Model file for the job. Use its own axes, mm. A direction names the side the tool comes from. Coordinates: 2 decimals unless noted, no trailing zeros. Put each result on its own line as item: value. Start each with the question number.
Q1. Drill centre lines: line 1 along Y through (x, z) = (12, 0.2); line 2 along Y through (x, z) = (-16, 1.3); line 3 along Z through (x, y) = (3, 4) (3 decimals). Where is each one in solid material? Low to high.
Q2. Cut at A-A (x = 0). Give the number of separate pieces and of enclosed holes in the cut face, then the cut area to 3 significant figures.
Q3. Drop flat-ended pins along their axis: pin 1 (0.9 mm diameter, centred on x = 0, y = 14.605, fed in from -Z); pin 2 (1.5 mm diameter, centred on y = -9, z = 0.5, fed in from +X); pin 3 (2 mm diameter, centred on x = 0, y = 6.985, fed in from -Z); pin 4 (5 mm diameter, centred on x = 6, y = 6.5, fed in from +Z) (3 decimals). Give the stop position or say it passes through.
Q4. Pull direction Y, two halves, no side cores. Call faces 6 (the cylindrical face through (-6.236, -0.098, 0.966)), 7 (the flat face through (-22.187, 0, 1)), 8 (the flat face through (0, -22.187, 1)): pulls with the +Y half, pulls with the -Y half, needs draft (parallel to the pull), parting line crosses it, or undercut.
Q5. Which spindle directions (+Z, -Z, +X, -X, +Y, -Y) get a long thin tool onto all of the face, cutting with end or side? Do faces 1 (the cylindrical face through (-0.164, 10.263, 0.966)), 2 (the cylindrical face through (-2.835, 0.893, -1.49)), 3 (the flat face through (13, 3.904, 1)), 4 (the flat face through (-3.904, -13, 1)), 5 (the flat face through (13, -3.904, 1)). Say none if no direction does.
```python
from build123d import *

# Parameters (mm, degrees)
SKETCH1_W         = 44.3738
SKETCH1_H         = 44.3738
EXTRUDE1_DEPTH    = 1.905
SKETCH2_R         = 4.2291
SKETCH2_R_2       = 2.9718
EXTRUDE2_DEPTH    = 3.0226
LPATTERN2_COUNT   = 5
LPATTERN2_PITCH   = 2.54
CIRPATTERN2_COUNT = 4
SKETCH6_W         = 18.282489336
SKETCH6_H         = 18.282489336
EXTRUDE3_DEPTH    = 5.9276
CIRPATTERN3_COUNT = 4


with BuildPart() as part:
    # Sketch1 → Extrude1 (new body)
    with BuildSketch(Plane.XY):
        Rectangle(SKETCH1_W, SKETCH1_H)
    extrude(amount=EXTRUDE1_DEPTH)

    # Sketch2 → Extrude2 (add)
    with BuildSketch(Plane(origin=(0, 0, 0), x_dir=(-1, 0, 0), z_dir=(0, 0, -1))):
        Circle(SKETCH2_R)
        Circle(SKETCH2_R_2, mode=Mode.SUBTRACT)
    extrude(amount=EXTRUDE2_DEPTH)

    # Sketch4 → #53 (0.0595) Diameter Hole1 (revolve, cut)
    with BuildSketch(Plane(origin=(6.985, 0, 1.905), x_dir=(0, -1, 0), z_dir=(1, 0, 0))):
        Polygon((0, 0), (0, 5.534040327), (0.75565, 5.08), (0.75565, 0), align=None)
    f_53_0_0595_diameter_hole1 = revolve(axis=Axis((6.985, 0, 8.255), (0, 0, -1)), mode=Mode.SUBTRACT)

    # LPattern2: #53 (0.0595) Diameter Hole1 ×5
    with Locations(*[(i * LPATTERN2_PITCH, 0, 0) for i in range(1, LPATTERN2_COUNT)]):
        add(f_53_0_0595_diameter_hole1, mode=Mode.SUBTRACT)

    # CirPattern2: #53 (0.0595) Diameter Hole1 ×4 about axis
    cirpattern2_axis = Axis((0, 0, 0), (0, 0, 1))
    for i in range(1, CIRPATTERN2_COUNT):
        add(f_53_0_0595_diameter_hole1.rotate(cirpattern2_axis, i * 360 / CIRPATTERN2_COUNT), mode=Mode.SUBTRACT)

    # CirPattern2 copy 1 sketch → CirPattern2 copy 1 (revolve, cut)
    with BuildSketch(Plane(origin=(0, 9.525, 1.905), x_dir=(1, 0, 0), z_dir=(0, 1, 0))):
        Polygon((0, 0), (0, 5.534040327), (0.75565, 5.08), (0.75565, 0), align=None)
    revolve(axis=Axis((0, 9.525, 8.255), (0, 0, -1)), mode=Mode.SUBTRACT)

    # CirPattern2 copy 2 sketch → CirPattern2 copy 2 (revolve, cut)
    with BuildSketch(Plane(origin=(-9.525, 0, 1.905), x_dir=(0, 1, 0), z_dir=(-1, 0, 0))):
        Polygon((0, 0), (0, 5.534040327), (0.75565, 5.08), (0.75565, 0), align=None)
    revolve(axis=Axis((-9.525, 0, 8.255), (0, 0, -1)), mode=Mode.SUBTRACT)

    # CirPattern2 copy 3 sketch → CirPattern2 copy 3 (revolve, cut)
    with BuildSketch(Plane(origin=(0, -9.525, 1.905), x_dir=(-1, 0, 0), z_dir=(0, -1, 0))):
        Polygon((0, 0), (0, 5.534040327), (0.75565, 5.08), (0.75565, 0), align=None)
    revolve(axis=Axis((0, -9.525, 8.255), (0, 0, -1)), mode=Mode.SUBTRACT)

    # CirPattern2 copy 4 sketch → CirPattern2 copy 4 (revolve, cut)
    with BuildSketch(Plane(origin=(0, 12.065, 1.905), x_dir=(1, 0, 0), z_dir=(0, 1, 0))):
        Polygon((0, 0), (0, 5.534040327), (0.75565, 5.08), (0.75565, 0), align=None)
    revolve(axis=Axis((0, 12.065, 8.255), (0, 0, -1)), mode=Mode.SUBTRACT)

    # CirPattern2 copy 5 sketch → CirPattern2 copy 5 (revolve, cut)
    with BuildSketch(Plane(origin=(-12.065, 0, 1.905), x_dir=(0, 1, 0), z_dir=(-1, 0, 0))):
        Polygon((0, 0), (0, 5.534040327), (0.75565, 5.08), (0.75565, 0), align=None)
    revolve(axis=Axis((-12.065, 0, 8.255), (0, 0, -1)), mode=Mode.SUBTRACT)

    # CirPattern2 copy 6 sketch → CirPattern2 copy 6 (revolve, cut)
    with BuildSketch(Plane(origin=(0, -12.065, 1.905), x_dir=(-1, 0, 0), z_dir=(0, -1, 0))):
        Polygon((0, 0), (0, 5.534040327), (0.75565, 5.08), (0.75565, 0), align=None)
    revolve(axis=Axis((0, -12.065, 8.255), (0, 0, -1)), mode=Mode.SUBTRACT)

    # CirPattern2 copy 7 sketch → CirPattern2 copy 7 (revolve, cut)
    with BuildSketch(Plane(origin=(0, 14.605, 1.905), x_dir=(1, 0, 0), z_dir=(0, 1, 0))):
        Polygon((0, 0), (0, 5.534040327), (0.75565, 5.08), (0.75565, 0), align=None)
    revolve(axis=Axis((0, 14.605, 8.255), (0, 0, -1)), mode=Mode.SUBTRACT)

    # CirPattern2 copy 8 sketch → CirPattern2 copy 8 (revolve, cut)
    with BuildSketch(Plane(origin=(-14.605, 0, 1.905), x_dir=(0, 1, 0), z_dir=(-1, 0, 0))):
        Polygon((0, 0), (0, 5.534040327), (0.75565, 5.08), (0.75565, 0), align=None)
    revolve(axis=Axis((-14.605, 0, 8.255), (0, 0, -1)), mode=Mode.SUBTRACT)

    # CirPattern2 copy 9 sketch → CirPattern2 copy 9 (revolve, cut)
    with BuildSketch(Plane(origin=(0, -14.605, 1.905), x_dir=(-1, 0, 0), z_dir=(0, -1, 0))):
        Polygon((0, 0), (0, 5.534040327), (0.75565, 5.08), (0.75565, 0), align=None)
    revolve(axis=Axis((0, -14.605, 8.255), (0, 0, -1)), mode=Mode.SUBTRACT)

    # CirPattern2 copy 10 sketch → CirPattern2 copy 10 (revolve, cut)
    with BuildSketch(Plane(origin=(0, 17.145, 1.905), x_dir=(1, 0, 0), z_dir=(0, 1, 0))):
        Polygon((0, 0), (0, 5.534040327), (0.75565, 5.08), (0.75565, 0), align=None)
    revolve(axis=Axis((0, 17.145, 8.255), (0, 0, -1)), mode=Mode.SUBTRACT)

    # CirPattern2 copy 11 sketch → CirPattern2 copy 11 (revolve, cut)
    with BuildSketch(Plane(origin=(-17.145, 0, 1.905), x_dir=(0, 1, 0), z_dir=(-1, 0, 0))):
        Polygon((0, 0), (0, 5.534040327), (0.75565, 5.08), (0.75565, 0), align=None)
    revolve(axis=Axis((-17.145, 0, 8.255), (0, 0, -1)), mode=Mode.SUBTRACT)

    # CirPattern2 copy 12 sketch → CirPattern2 copy 12 (revolve, cut)
    with BuildSketch(Plane(origin=(0, -17.145, 1.905), x_dir=(-1, 0, 0), z_dir=(0, -1, 0))):
        Polygon((0, 0), (0, 5.534040327), (0.75565, 5.08), (0.75565, 0), align=None)
    revolve(axis=Axis((0, -17.145, 8.255), (0, 0, -1)), mode=Mode.SUBTRACT)

    # Sketch6 → Extrude3 (cut, through all)
    with BuildSketch(Plane.XY.offset(1.905)):
        with Locations((-13.045655332, 13.045655332)):
            Rectangle(SKETCH6_W, SKETCH6_H)
    extrude3 = extrude(amount=-EXTRUDE3_DEPTH, mode=Mode.SUBTRACT)

    # CirPattern3: Extrude3 ×4 about axis
    cirpattern3_axis = Axis((0, 0, 0), (0, 0, 1))
    for i in range(1, CIRPATTERN3_COUNT):
        add(extrude3.rotate(cirpattern3_axis, i * 360 / CIRPATTERN3_COUNT), mode=Mode.SUBTRACT)


solid = part.part
```
Computed values:
1. line 1: -3.9 to -0.75, 0.75 to 3.9
1. line 2: -3.9 to 3.9
1. line 3: 0 to 1.905
2. separate pieces: 11
2. enclosed holes: 0
2. area: 63.3 mm2
3. pin 1: through
3. pin 2: x = 3.9
3. pin 3: z = 0
3. pin 4: z = 1.905
4. face 6: undercut
4. face 7: needs draft
4. face 8: pulls with the -Y half
5. face 1: +Z, -Z
5. face 2: -Z
5. face 3: +Z, -Z, +X, +Y
5. face 4: +Z, -Z, -X, -Y
5. face 5: +Z, -Z, +X, -Y
